The model under review builds one solid part; all positions refer to its coordinate system, in mm. A direction names the side the tool comes from. Round coordinates to 2 decimals unless told otherwise and drop trailing zeros. Order: outer loops, then holes, each group sorted by start corner. A loop starts at its lowest first (then second) coordinate and runs counter-clockwise, first axis right, second up. Notation, with made-up numbers: M 44.5,53 L 101.5,53 A23 ccw 101.5,67 Z; hole C 79,75.25 d8. An arc over 180 degrees is marked long. Answer as a JSON object with one key per item and string values. Group by question number.
1. Mouldability with a two-part tool opening along Z and no side actions: class faces 1 (the face through (2.53, 1.51, 4.73)), 2 (the face through (8, -0.5, 6)) as released by +Z, released by -Z, zero draft, split by the parting line, or undercut.
2. Clearance check with flat-ended pins moving along their axes: P1, Ø3, axis at x = 9.5, y = -3, coming from the +Z side; P2, Ø3, axis at x = 12.25, z = 5, coming from the +Y side; P3, Ø4, axis at x = 3, z = 4, coming from the +Y side; P4, Ø8, axis at y = 2.5, z = 0.5, coming from the +X side. State where each tip first meets the part, or that it passes through.
3. Add section C-C on y = 1.75. Give the number of separate pieces and of enclosed holes in the cut face, and give its area (3 significant figures).
4. Machinability: for faces 3 (the face through (2.7, 2.5, 6)), 4 (the face through (7.5, 4, 0)), 5 (the face through (3.8, -3.01, 3.75)), 6 (the face through (12.2, 0.5, -3.5)), 7 (the face through (4, 3, 0)), which of the approach directions +Z, -Z, +X, -X, +Y, -Y give a long, thin tool a straight path to every point of the face, cutting with its end or side? Answer none if there is none.
5. To check wall thickness, follow probe 1 along X at (y, z) = (1.7, 5); probe 2 along X at (y, z) = (-4.25, 5); probe 3 along X at (y, z) = (3.5, -3). State the ranges of each line that lie inside material, in increasing order. Write a range as [from, to].
6. Add section A-A on z = 0. State the section outline as (x, y) points.
7. Add section B-B on x = 3.75. State the section outline as (y, z) points.
Autodesk Inventor part; units mm, degrees
ref_plane "L_XY" through (3.75, 2.5, 5) normal (0, 1, 0) x (1, 0, 0)
ref_plane "L_YZ" through (3.75, 2.5, 5) normal (1, 0, 0) x (0, 0, -1)
ref_plane "L_ZX" through (3.75, 2.5, 5) normal (0, 0, -1) x (0, 1, 0)
sketch "Sketch_1" plane through (0, 0, 0) normal (0, 0, 1) x (1, 0, 0)
  line L0 (16, 0) -> (0, 0)
  line L1 (0, 3) -> (7.5, 3)
  line L2 (7.5, 3) -> (7.5, 3.1)
  line L3 (7.5, 3.1) -> (8.5, 3.1)
  line L4 (8.5, 3.1) -> (8.5, 3)
  line L5 (8.5, 3) -> (16, 3)
  line L6 (16, 3) -> (16, 7.75)
  line L7 (16, 7.75) -> (15.75, 8)
  line L8 (15.75, 8) -> (0.25, 8)
  line L9 (0.25, 8) -> (0, 7.75)
  line L10 (0, 7.75) -> (0, 3)
revolve "Revolution1" add sketch "Sketch_1" angle 360 about axis through (16, 0, 0) along (1, 0, 0)
sketch "Sketch_2" plane through (0, 0, 0) normal (1, 0, 0) x (0, 1, 0)
  line L0 (0.5, 8) -> (-0.5, 8)
  line L1 (-0.5, 8) -> (-0.5, -4)
  line L2 (-0.5, -4) -> (0.5, -4)
  line L3 (0.5, -4) -> (0.5, 8)
extrude "Extrusion1" cut sketch "Sketch_2" along normal blind 16
sketch "Sketch_3" plane through (0, 0, 0) normal (0, 1, 0) x (-1, 0, 0)
  line L0 (-8.5, 0) -> (-7.5, 0)
  line L1 (-7.5, 0) -> (-7.5, -8)
  line L2 (-7.5, -8) -> (-8.5, -8)
  line L3 (-8.5, -8) -> (-8.5, 0)
  line L4 (-8.5, 0) -> (-7.5, 0)
revolve "Revolution2" cut sketch "Sketch_3" angle 180 about axis through (8.5, 0, 0) along (1, 0, 0)
sketch "Sketch_4" plane through (3.75, 0, 0) normal (1, 0, 0) x (0, 0, -1)
  line L0 (-5, 8) -> (-5, -8)
  line L1 (-5, -8) -> (-6.25, -8)
  line L2 (-6.25, -8) -> (-6.25, 2.5)
  line L3 (-6.25, 2.5) -> (-7.4, 2.5)
  line L4 (-7.4, 2.5) -> (-7.4, 8)
  line L5 (-7.4, 8) -> (-5, 8)
  line L6 (-5, 8) -> (-5, -8)
revolve "Revolution3" cut sketch "Sketch_4" angle 360 about axis through (3.75, 8, 5) along (0, 1, 0)
sketch "Sketch_5" plane through (12.25, 0, 0) normal (1, 0, 0) x (0, 0, -1)
  line L0 (-5, 8) -> (-5, -8)
  line L1 (-5, -8) -> (-6.25, -8)
  line L2 (-6.25, -8) -> (-6.25, 2.5)
  line L3 (-6.25, 2.5) -> (-7.4, 2.5)
  line L4 (-7.4, 2.5) -> (-7.4, 8)
  line L5 (-7.4, 8) -> (-5, 8)
  line L6 (-5, 8) -> (-5, -8)
revolve "Revolution4" cut sketch "Sketch_5" angle 360 about axis through (12.25, 8, 5) along (0, 1, 0)
ref_plane "L_XY" through (3.75, 2.5, 5) normal (0, 1, 0) x (1, 0, 0)
ref_plane "L_YZ" through (3.75, 2.5, 5) normal (1, 0, 0) x (0, 0, -1)
ref_plane "L_ZX" through (3.75, 2.5, 5) normal (0, 0, -1) x (0, 1, 0)
ref_plane "R_XY" through (12.25, 2.5, 5) normal (0, 1, 0) x (1, 0, 0)
ref_plane "R_YZ" through (12.25, 2.5, 5) normal (1, 0, 0) x (0, 0, -1)
ref_plane "R_ZX" through (12.25, 2.5, 5) normal (0, 0, -1) x (0, 1, 0)
properties part number "D_CPRC16-6-6" material "鋼、炭素鋼"
Recorded:
{
 "1": {"face 1": "undercut", "face 2": "zero draft"},
 "2": {"P1": "stops at z = 7.86", "P2": "stops at y = 2.5", "P3": "stops at y = 7.75", "P4": "stops at x = 16"},
 "3": {"separate pieces": "4", "enclosed holes": "2", "area": "151 mm²"},
 "4": {"face 3": "+Y", "face 4": "+Z, -Z, +Y", "face 5": "+Y, -Y", "face 6": "+Z, +X, -X", "face 7": "+X, -X"},
 "5": {"probe 1": "x = [0, 2.5], [5, 7.5], [8.5, 11], [13.5, 16]", "probe 2": "x = [0, 2.5], [5, 11], [13.5, 16]", "probe 3": "x = [0, 7.5], [8.5, 16]"},
 "6": {"outline": "M 0,-7.75 L 0.25,-8 L 15.75,-8 L 16,-7.75 L 16,-3 L 8.5,-3 L 8.5,-3.1 L 7.5,-3.1 L 7.5,-3 L 0,-3 Z; M 0,3 L 7.5,3 L 7.5,8 L 0.25,8 L 0,7.75 Z; M 8.5,3 L 16,3 L 16,7.75 L 15.75,8 L 8.5,8 Z"},
 "7": {"outline": "M -7.07,3.75 A8 ccw long 7.57,2.6 L 2.5,2.6 L 2.5,3.75 L 0.5,3.75 L 0.5,2.96 A3 cw 0.5,-2.96 L 0.5,-4 L -0.5,-4 L -0.5,-2.96 A3 cw -0.5,2.96 L -0.5,3.75 Z; M -4.99,6.25 L -0.5,6.25 L -0.5,7.98 A8 ccw Z; M 0.5,6.25 L 2.5,6.25 L 2.5,7.4 L 3.04,7.4 A8 ccw 0.5,7.98 Z"}
}
